Read the model definition and answer for the solid it produces. Units are mm, in the model's axes. A direction names the side the tool comes from. Give positions to 0.01 mm unless a question says otherwise; leave off trailing zeros. Order: outer loops, then holes, each group sorted by start corner. A loop starts at its lowest first (then second) coordinate and runs counter-clockwise, first axis right, second up. Notation, with made-up numbers: (60, -5) - (93, -5) arc R27 ccw to (93, 33) - close; hole circle Ø6 at (66.25, 56.25). An arc over 180 degrees is marked (long way). Use a Markdown table: item, result. Add a question column.
1. Which of the six approach directions +Z, -Z, +X, -X, +Y, -Y give full straight-line access (tool end or side, diameter ignored) to faces 5 (the flat face through (-25, -6.35, 0)), 6 (the flat face through (-22, 0, 20)), 7 (the flat face through (0, -6.35, -25))?
2. Flat-ended cylindrical pins translate along their axes: P1, Ø1, axis at y = -5.5, z = -25, coming from the +X side; P2, Ø6, axis at y = -7.5, z = -13, coming from the -X side; P3, Ø3, axis at x = 0.5, z = -31, coming from the +Y side. Find the tip coordinate at first contact, or state that the pin passes through.
3. For a pull along X with two mould halves and no side action, classify faces 1 (the flat face through (22, 0, -20)), 2 (the flat face through (11, -5.08, 15)), 3 (the cylindrical face through (36.34, -5.01, 11.44)), 4 (the flat face through (-12.7, -3, -23)) as released by +X, released by -X, zero draft, split by the parting line, or undercut.
4. A cutting plane is placed at D-D on z = -23.5. Determine the outline of the cut face in (x, y).
5. Consider L1, parallel to Z at x = 0, y = -8.55; L2, parallel to Y at x = 2.5, z = -17. Determine where each line is inside the solid, lowest interval first.
6. A cutting plane is placed at A-A on x = 0. Determine the outline of the cut face in (y, z), and give its area (3 significant figures).
7. A cutting plane is placed at C-C on y = -3. Determine the outline of the cut face in (x, z).
8. A cutting plane is placed at B-B on z = 0. Determine the outline of the cut face in (x, y), and give its area (3 significant figures).
```python
from build123d import *

# Parameters (mm, degrees)
F0_R          = 12.7
F1_DEPTH      = 17.78
F2_R          = 38.1
F3_DEPTH      = 10.16
F4_R          = 12.954
F5_DEPTH      = 17.781
F5_DEPTH_BACK = 115
F6_W          = 5.08
F6_H          = 20.32
F7_DEPTH      = 38.101
F7_DEPTH_BACK = 38.101
F8_W          = 25.4
F8_H          = 5.08
F9_DEPTH      = 38.101
F9_DEPTH_BACK = 38.101
F11_DEPTH     = 6.35


# Not quite as in the source:
# - an extrude ends at something that could not be found from the text; its depth is read off the source's solid


with BuildPart() as f1:
    # F0 (on Front) → F1 (new body)
    with BuildSketch(Plane.XZ):
        Circle(F0_R)
    extrude(amount=F1_DEPTH)

    # F2 (on Front) → F3 (join)
    with BuildSketch(Plane.XZ):
        Circle(F2_R)
    extrude(amount=F3_DEPTH)

    # F4 (on Front) → F5 (cut, two sides)
    with BuildSketch(Plane.XZ) as f5_sk:
        Circle(F4_R)
    extrude(amount=F5_DEPTH, mode=Mode.SUBTRACT)
    extrude(f5_sk.sketch, amount=-F5_DEPTH_BACK, mode=Mode.SUBTRACT)

    # F6 (on Right) → F7 (cut, two sides)
    with BuildSketch(Plane.YZ) as f7_sk:
        with Locations((-2.54, 0)):
            Rectangle(F6_W, F6_H)
    extrude(amount=F7_DEPTH, mode=Mode.SUBTRACT)
    extrude(f7_sk.sketch, amount=-F7_DEPTH_BACK, mode=Mode.SUBTRACT)

    # F8 (on Top) → F9 (cut, two sides)
    with BuildSketch(Plane.XY) as f9_sk:
        with Locations((0, -2.54)):
            Rectangle(F8_W, F8_H)
    extrude(amount=-F9_DEPTH, mode=Mode.SUBTRACT)
    extrude(f9_sk.sketch, amount=F9_DEPTH_BACK, mode=Mode.SUBTRACT)

    # F10 (on face) → F11 (cut)
    with BuildSketch(Plane(origin=(0, 0, 0), x_dir=(-1, 0, 0), z_dir=(0, 1, 0))):
        with BuildLine():
            Line((1.27, -1.27), (38.0788274504, -1.27))
            ThreePointArc((38.0788274504, -1.27), (38.1, 0), (38.0788274504, 1.27))
            Line((38.0788274504, 1.27), (1.27, 1.27))
            Line((1.27, 1.27), (1.27, 38.0788274504))
            ThreePointArc((1.27, 38.0788274504), (0, 38.1), (-1.27, 38.0788274504))
            Line((-1.27, 38.0788274504), (-1.27, 1.27))
            Line((-1.27, 1.27), (-38.0788274504, 1.27))
            ThreePointArc((-38.0788274504, 1.27), (-38.1, 0), (-38.0788274504, -1.27))
            Line((-38.0788274504, -1.27), (-1.27, -1.27))
            Line((-1.27, -1.27), (-1.27, -38.0788274504))
            ThreePointArc((-1.27, -38.0788274504), (0, -38.1), (1.27, -38.0788274504))
            Line((1.27, -38.0788274504), (1.27, -1.27))
        make_face()
    extrude(amount=-F11_DEPTH, mode=Mode.SUBTRACT)


solid = f1.part
```
Output values:
| question | item | result |
|---|---|---|
| 1 | face 5 | +X, -X, +Y |
| 1 | face 6 | +Z, -Z, +X, -X, +Y |
| 1 | face 7 | +Z, -Z, +Y |
| 2 | P1 | x = 29.18 |
| 2 | P2 | x = -36.76 |
| 2 | P3 | y = -5.08 |
| 3 | face 1 | zero draft |
| 3 | face 2 | undercut |
| 3 | face 3 | split by the parting line |
| 3 | face 4 | undercut |
| 4 | outline | (-29.99, -10.16) - (29.99, -10.16) - (29.99, 0) - (12.7, 0) - (12.7, -5.08) - (1.27, -5.08) - (1.27, -6.35) - (-1.27, -6.35) - (-1.27, -5.08) - (-12.7, -5.08) - (-12.7, 0) - (-29.99, 0) - close |
| 5 | L1 | -38.1 to -12.95, 12.95 to 38.1 |
| 5 | L2 | -10.16 to -5.08 |
| 6 | outline | (-10.16, -38.1) - (-6.35, -38.1) - (-6.35, -12.95) - (-10.16, -12.95) - close; (-10.16, 12.95) - (-6.35, 12.95) - (-6.35, 38.1) - (-10.16, 38.1) - close |
| 6 | area | 192 mm² |
| 7 | outline | (-36.72, -10.16) arc R38.1 ccw to (-12.7, -35.92) - (-12.7, -10.16) - close; (-36.72, 10.16) - (-12.7, 10.16) - (-12.7, 35.92) arc R38.1 ccw to start; (12.7, -35.92) arc R38.1 ccw to (36.72, -10.16) - (12.7, -10.16) - close; (12.7, 10.16) - (36.72, 10.16) arc R38.1 ccw to (12.7, 35.92) - close |
| 8 | outline | (-38.1, -10.16) - (-12.95, -10.16) - (-12.95, -6.35) - (-38.1, -6.35) - close; (12.95, -10.16) - (38.1, -10.16) - (38.1, -6.35) - (12.95, -6.35) - close |
| 8 | area | 192 mm² |
